```python
from build123d import *

# Parameters (mm, degrees)
SKETCH1_R           = 9
BOSS_EXTRUDE1_DEPTH = 8
SKETCH2_R           = 9
BOSS_EXTRUDE2_DEPTH = 2
SKETCH3_R           = 3
CUT_EXTRUDE1_DEPTH  = 17.186414056
FILLET3_R           = 0.5
SKETCH4_R           = 1.75
CUT_EXTRUDE2_DEPTH  = 8
SKETCH5_R           = 2
CUT_EXTRUDE3_DEPTH  = 2


with BuildPart() as part:
    # Sketch1 → Boss-Extrude1 (new body)
    with BuildSketch(Plane(origin=(0, 0, 0), x_dir=(0, 0, -1), z_dir=(1, 0, 0))):
        Circle(SKETCH1_R)
        with BuildLine():
            ThreePointArc((1.704, 1.690084022), (0, 2.4), (-1.704, 1.690084022))
            ThreePointArc((-1.704, 1.690084022), (-3, 0), (-1.704, -1.690084022))
            ThreePointArc((-1.704, -1.690084022), (0, -2.4), (1.704, -1.690084022))
            ThreePointArc((1.704, -1.690084022), (3, 0), (1.704, 1.690084022))
        make_face(mode=Mode.SUBTRACT)
    extrude(amount=BOSS_EXTRUDE1_DEPTH)

    # Sketch2 → Boss-Extrude2 (add)
    with BuildSketch(Plane(origin=(8, 0, 0), x_dir=(0, 0, -1), z_dir=(1, 0, 0))):
        Circle(SKETCH2_R)
    extrude(amount=BOSS_EXTRUDE2_DEPTH)

    # Sketch3 → Cut-Extrude1 (cut, through all)
    with BuildSketch(Plane(origin=(10, 0, 0), x_dir=(0, 0, -1), z_dir=(1, 0, 0))):
        with Locations((-4.400859472, 10.624614624)):
            Circle(SKETCH3_R)
        with Locations((4.400859472, 10.624614624)):
            Circle(SKETCH3_R)
        with Locations((10.624614624, 4.400859472)):
            Circle(SKETCH3_R)
        with Locations((4.400859472, -10.624614624)):
            Circle(SKETCH3_R)
        with Locations((-10.624614624, -4.400859472)):
            Circle(SKETCH3_R)
        with Locations((-10.624614624, 4.400859472)):
            Circle(SKETCH3_R)
        with Locations((-4.400859472, -10.624614624)):
            Circle(SKETCH3_R)
        with Locations((10.624614624, -4.400859472)):
            Circle(SKETCH3_R)
    extrude(amount=-CUT_EXTRUDE1_DEPTH, mode=Mode.SUBTRACT)

    # Fillet3
    fillet3_edges = [part.edges().sort_by_distance(p)[0] for p in [
        (5, 8.763991921, 2.047546243),
        (5, 7.64491195, 4.749244284),
        (5, 2.047546243, -8.763991921),
        (5, 4.749244284, -7.64491195),
        (5, -8.763991921, -2.047546243),
        (5, -7.64491195, -4.749244284),
        (5, -2.047546243, 8.763991921),
        (5, -4.749244284, 7.64491195),
        (5, 7.64491195, -4.749244284),
        (5, 8.763991921, -2.047546243),
        (5, 4.749244284, 7.64491195),
        (5, 2.047546243, 8.763991921),
        (5, -7.64491195, 4.749244284),
        (5, -8.763991921, 2.047546243),
        (5, -4.749244284, -7.64491195),
        (5, -2.047546243, -8.763991921),
    ]]
    fillet(fillet3_edges, radius=FILLET3_R)

    # Sketch4 → Cut-Extrude2 (cut)
    with BuildSketch(Plane.ZY):
        with Locations((0, 5.5)):
            Circle(SKETCH4_R)
    extrude(amount=-CUT_EXTRUDE2_DEPTH, mode=Mode.SUBTRACT)

    # Sketch5 → Cut-Extrude3 (cut)
    with BuildSketch(Plane.ZY):
        with Locations((0, 5.5)):
            Circle(SKETCH5_R)
    extrude(amount=-CUT_EXTRUDE3_DEPTH, mode=Mode.SUBTRACT)


solid = part.part
```
Can you work these out from the model? Positions are in its coordinate system, mm. A direction names the side the tool comes from. Round coordinates to 2 decimals unless told otherwise and drop trailing zeros. Loops run counter-clockwise (first coordinate to the right, second up) from the corner with the lowest first, then second, coordinate; pieces in that order, holes last. Notation, with made-up numbers: (35, 26.25) -> (70, 26.25) arc R11 cw to (70, 32.25) -> close; hole circle Ø2 at (45, -13.5). An arc over 180 degrees is marked (long way). One line per item, written item: value. Start each with the question number.
1. If we section it at D-D, the plane y = -7.25: Write out the boundary of the cut face in (x, z), then the cut area to 3 significant figures.
2. If we mould it in two halves opening along Z, with no side actions, what happens to faces 1 (the cylindrical face through (4.93, -6.38, -6.35)), 2 (the cylindrical face through (4, 0, -3)), 3 (the cylindrical face through (5.07, -3.271, 7.846))? For each: pulls with the +Z half, pulls with the -Z half, needs draft (parallel to the pull), parting line crosses it, or undercut.
3. If we section it at C-C, the plane x = 0.75: Give the number of separate pieces and of enclosed holes in the cut face, then the cut area to 3 significant figures.
4. If we section it at B-B, the plane y = 4: Write out the boundary of the cut face in (x, z), then the cut area to 3 significant figures.
5. If I drill on probe 1 along Y at (x, z) = (0.8, 0); probe 2 along Y at (x, z) = (6.75, 1); probe 3 along X at (y, z) = (1.5, -1.75), over which ranges is the centre line in solid material (lowest first)?
6. For pin 1 (1.8 mm diameter, centred on y = 5, z = 0, fed in from -X); pin 2 (2 mm diameter, centred on x = 8, z = 2, fed in from +Y); pin 3 (5 mm diameter, centred on x = 2, z = -5.5, fed in from -Y), each with a flat end and sliding along its axis, tell me the tip position at first contact or that it passes through.
7. For faces 4 (the cylindrical face through (5, 0, -9)), 5 (the flat face through (8, 6, 0)), which set-ups out of +Z, -Z, +X, -X, +Y, -Y let a thin tool reach every point of the face, with its end or its side?
8. If we section it at A-A, the plane z = 0: Write out the boundary of the cut face in (x, y).
Calculated:
1. outline: (0, -5.33) -> (10, -5.33) -> (10, 5.33) -> (0, 5.33) -> close
1. area: 107 mm²
2. face 1: pulls with the -Z half
2. face 2: undercut
2. face 3: pulls with the +Z half
3. separate pieces: 1
3. enclosed holes: 2
3. area: 213 mm²
4. outline: (0, -7.65) -> (10, -7.65) -> (10, 7.65) -> (0, 7.65) -> (0, 1.32) -> (2, 1.32) -> (2, 0.9) -> (8, 0.9) -> (8, -0.9) -> (2, -0.9) -> (2, -1.32) -> (0, -1.32) -> close
4. area: 137 mm²
5. probe 1: y = -9 to -2.4, 2.4 to 3.5, 7.5 to 9
5. probe 2: y = -8.94 to -2.18, 2.18 to 4.06, 6.94 to 8.94
5. probe 3: x = 8 to 10
6. pin 1: stops at x = 8
6. pin 2: stops at y = 8.94
6. pin 3: stops at y = -7.97
7. face 4: -Z, +X, -X
7. face 5: -X
8. outline: (0, -9) -> (10, -9) -> (10, 9) -> (0, 9) -> (0, 7.5) -> (2, 7.5) -> (2, 7.25) -> (8, 7.25) -> (8, 3.75) -> (2, 3.75) -> (2, 3.5) -> (0, 3.5) -> (0, 2.4) -> (8, 2.4) -> (8, -2.4) -> (0, -2.4) -> close
